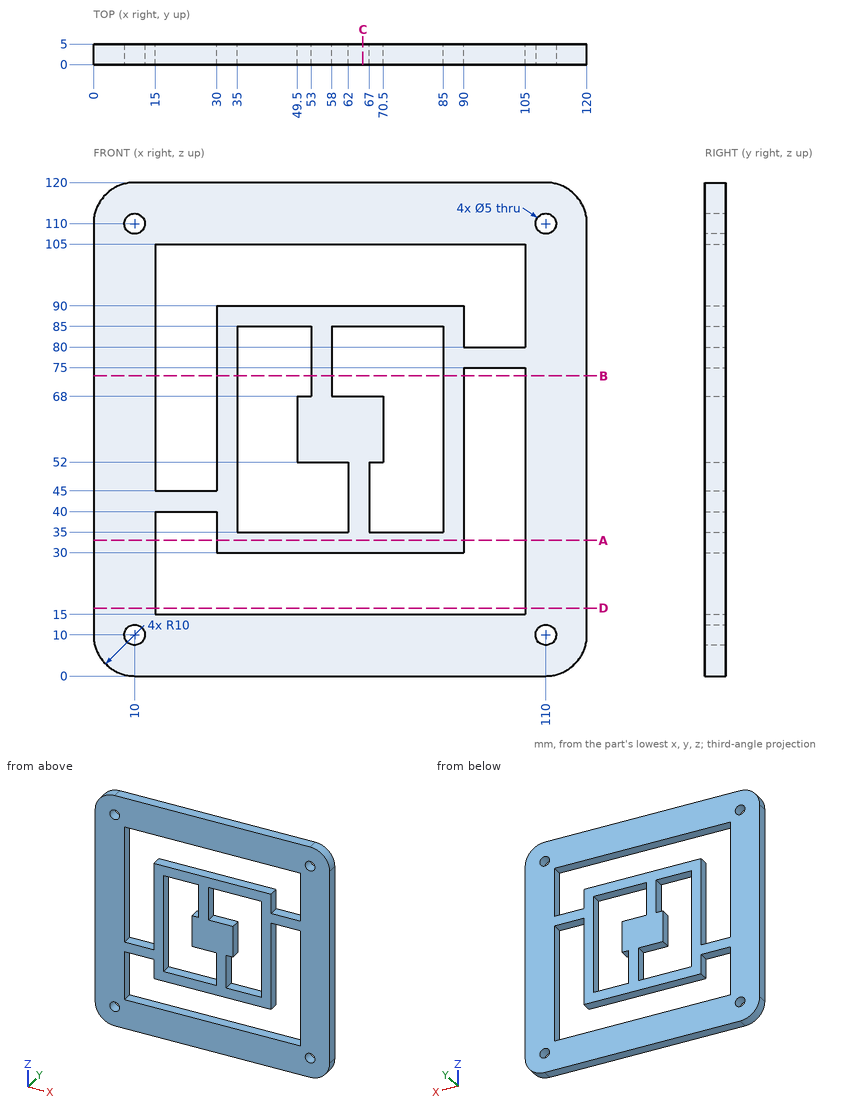
Check sheet for the drawn part. Datum: minimum x, y, z corner. Units: mm. Coordinates: 2 decimals unless noted, no trailing zeros. Write each loop counter-clockwise with the first axis right and the second up, starting at its lowest first coordinate (ties: lowest second). Pieces come first, ordered by that corner, then holes. Notation, with made-up numbers: (9.5, 78.25) - (43.5, 78.25) arc R25 ccw to (43.5, 100.25) - close; hole circle Ø5 at (53.5, 29.25). An arc over 180 degrees is marked (long way). Answer as a JSON object with one key per item and string values.
(1) Thickness scan on line 1 along Z through (x, y) = (110, 1.3); line 2 along X through (y, z) = (2.95, 66). Record the ranges inside material, lowest first.
Report:
{"line 1": "0 to 7.5, 12.5 to 107.5, 112.5 to 120", "line 2": "0 to 15, 30 to 35, 49.5 to 70.5, 85 to 90, 105 to 120"}
(2) Cross-section at D-D on z = 16.5. Record the cut outline in (x, y).
Report:
{"outline": "(0, 0) - (15, 0) - (15, 5) - (0, 5) - close; (105, 0) - (120, 0) - (120, 5) - (105, 5) - close"}
(3) Cross-section at C-C on x = 65.5. Record the cut outline in (y, z), plus the area to 3 significant figures.
Report:
{"outline": "(0, 0) - (5, 0) - (5, 15) - (0, 15) - close; (0, 30) - (5, 30) - (5, 68) - (0, 68) - close; (0, 85) - (5, 85) - (5, 90) - (0, 90) - close; (0, 105) - (5, 105) - (5, 120) - (0, 120) - close", "area": "365 mm^2"}
(4) Cross-section at A-A on z = 33. Record the cut outline in (x, y).
Report:
{"outline": "(0, 0) - (15, 0) - (15, 5) - (0, 5) - close; (30, 0) - (90, 0) - (90, 5) - (30, 5) - close; (105, 0) - (120, 0) - (120, 5) - (105, 5) - close"}
(5) Cross-section at B-B on z = 73. Record the cut outline in (x, y), plus the area to 3 significant figures.
Report:
{"outline": "(0, 0) - (15, 0) - (15, 5) - (0, 5) - close; (30, 0) - (35, 0) - (35, 5) - (30, 5) - close; (53, 0) - (58, 0) - (58, 5) - (53, 5) - close; (85, 0) - (90, 0) - (90, 5) - (85, 5) - close; (105, 0) - (120, 0) - (120, 5) - (105, 5) - close", "area": "225 mm^2"}
